Here's the drawing with two shaded views (mm, measured from the low corner). I have some questions. A direction names the side the tool comes from. Round coordinates to 2 decimals unless told otherwise and drop trailing zeros. Write each loop counter-clockwise with the first axis right and the second up, starting at its lowest first coordinate (ties: lowest second). Pieces come first, ordered by that corner, then holes.
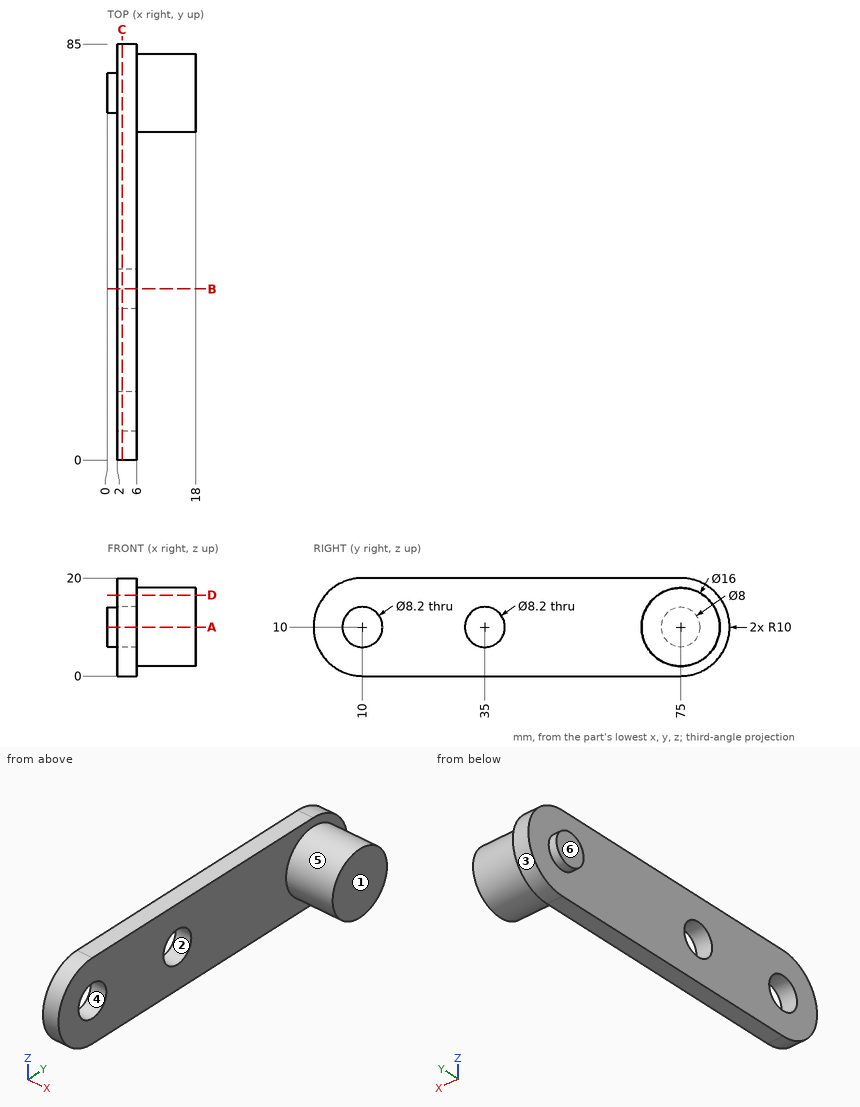
Q1. I'm going to push flat-ended pins straight in: pin 1 Ø12 at (y, z) = (58, 6) entering from -X; pin 2 Ø3 at (y, z) = (41.5, 7) entering from +X; pin 3 Ø3 at (x, z) = (14.5, 7) entering from -Y; pin 4 Ø6.5 at (y, z) = (35, 10) entering from -X. Where does each tip first touch, or does it pass through?
Q2. Imagine slicing it at B-B, the plane y = 35. Write out the boundary of the cut face in (x, z), then the cut area to 3 significant figures.
Q3. Imagine slicing it at C-C, the plane x = 3. Write out the boundary of the cut face in (y, z).
Q4. If I drill on L1, parallel to Z at x = 3.8, y = 35; L2, parallel to X at y = 66, z = 5.75; L3, parallel to X at y = 72.5, z = 3, over which ranges is the centre line in solid material (lowest first)?
Q5. Imagine slicing it at A-A, the plane z = 10. Write out the boundary of the cut face in (x, y), then the cut area to 3 significant figures.
Q6. Imagine slicing it at D-D, the plane z = 16.5. Write out the boundary of the cut face in (x, y), then the cut area to 3 significant figures.
Q7. We'd pull the mould along Z, two halves only. Please class the marked faces 1, 2, 3 and 4: pulls with the +Z half, pulls with the -Z half, needs draft (parallel to the pull), parting line crosses it, or undercut.
Q8. On a 3-axis mill with a long thin cutter (end or side, diameter ignored), from which of +Z, -Z, +X, -X, +Y, -Y can I reach the whole of each face in a straight line? I mean the marked faces 5 and 6. Say none if no direction works.
Results found:
1. pin 1: stops at x = 2
1. pin 2: stops at x = 6
1. pin 3: stops at y = 67.14
1. pin 4: passes through
2. outline: (2, 0) - (6, 0) - (6, 5.9) - (2, 5.9) - close; (2, 14.1) - (6, 14.1) - (6, 20) - (2, 20) - close
2. area: 47.2 mm2
3. outline: (10, 0) - (75, 0) arc R10 ccw to (75, 20) - (10, 20) arc R10 ccw to start; hole circle Ø8.2 at (10, 10); hole circle Ø8.2 at (35, 10)
4. L1: z = 0 to 5.9, 14.1 to 20
4. L2: x = 2 to 6
4. L3: x = 2 to 18
5. outline: (0, 71) - (2, 71) - (2, 39.1) - (6, 39.1) - (6, 67) - (18, 67) - (18, 83) - (6, 83) - (6, 85) - (2, 85) - (2, 79) - (0, 79) - close; (2, 0) - (6, 0) - (6, 5.9) - (2, 5.9) - close; (2, 14.1) - (6, 14.1) - (6, 30.9) - (2, 30.9) - close
5. area: 482 mm2
6. outline: (2, 2.4) - (6, 2.4) - (6, 70.34) - (18, 70.34) - (18, 79.66) - (6, 79.66) - (6, 82.6) - (2, 82.6) - close
6. area: 433 mm2
7. face 1: needs draft
7. face 2: undercut
7. face 3: parting line crosses it
7. face 4: undercut
8. face 5: +X
8. face 6: +Z, -Z, -X, +Y, -Y
